Build history of the part. All positions in model axes, mm. A direction names the side the tool comes from. Give positions to 0.01 mm unless a question says otherwise; leave off trailing zeros. Order: outer loops, then holes, each group sorted by start corner. A loop starts at its lowest first (then second) coordinate and runs counter-clockwise, first axis right, second up. Notation, with made-up numbers: (21, -4) - (37, -4) arc R19 cw to (37, 8) - close; hole circle Ø3 at (69.5, 15.25). An arc over 180 degrees is marked (long way). Use a Markdown table: item, result.
Autodesk Fusion 360 part; units mm, degrees
sketch "スケッチ1" plane through (0, 0, 0) normal (0, 0, 1) x (1, 0, 0)
  line L0 (-9.5, 140) -> (-80.5, 140)
  line L1 (-80.5, 140) -> (-80.5, -140)
  line L2 (-80.5, -140) -> (-9.5, -140)
  line L3 (80.5, 20) -> (80.5, 130)
  line L4 (74.75, 130) -> (-80.5, -140) construction
  line L5 (-80.5, 140) -> (38.0073, -66.0997) construction
  line L6 (-9.5, 140) -> (-9.5, 130)
  line L7 (-9.5, 130) -> (80.5, 130)
  line L8 (-80.5, -140) -> (-9.5, -140) construction
  line L9 (80.5, 0) -> (-9.5, -140)
  line L10 (80.5, 0) -> (-9.5, 0)
  line L11 (-9.5, 0) -> (-9.5, 20)
  line L12 (-9.5, 20) -> (80.5, 20)
  dimension "d2" = 280
  dimension "d5" = 71
  dimension "d7" = 90
  dimension "d8" = 20
extrude "押し出し1" add sketch "スケッチ1" along normal blind 6
chamfer "面取り1" distance 25 angle 45 2 edges at (-80.5, -140, 3) (-80.5, 140, 3)
sketch "スケッチ2" plane through (0, 0, 6) normal (0, 0, 1) x (-1, 0, 0)
  line L0 (55.5, -140) -> (80.5, -115)
  line L1 (80.5, -115) -> (80.5, 115)
  line L2 (80.5, 115) -> (55.5, 140)
  line L3 (55.5, 140) -> (9.5, 140)
  line L4 (9.5, 140) -> (-80.5, 0)
  line L5 (-80.5, 0) -> (9.5, 0)
  line L6 (9.5, 0) -> (9.5, -20)
  line L7 (9.5, -20) -> (-80.5, -20)
  line L8 (-80.5, -20) -> (-80.5, -130)
  line L9 (-80.5, -130) -> (9.5, -130)
  line L10 (9.5, -130) -> (9.5, -140)
  line L11 (9.5, -140) -> (55.5, -140)
  line L12 (-80.5, -130) -> (-40.5, -130) construction
  line L13 (-40.5, -130) -> (-40.5, -100) construction
  line L14 (-40.5, -100) -> (-80.5, -100) construction
  line L15 (-80.5, -100) -> (-80.5, -130) construction
  line L16 (-40.5, -100) -> (-40.5, -50) construction
  point P0 (-40.5, -100)
  point P1 (-40.5, -50)
  dimension "d12" = 40
  dimension "d13" = 30
  dimension "d14" = 50
hole "穴1" at (40.5, 100, 6) at (40.5, 50, 6) direction (0, 0, -1) diameter 18 end through all
equation "d5 = 25 mm + 46 mm"
1) Slice it at A-A (y = 50). Write the cut outline in (x, z), and give its area (3 significant figures).
Computed:
| item | result |
|---|---|
| outline | (-80.5, 0) - (31.5, 0) - (31.5, 6) - (-80.5, 6) - close; (49.5, 0) - (80.5, 0) - (80.5, 6) - (49.5, 6) - close |
| area | 858 mm² |
2) Slice it at C-C (z = 4.9). Write the cut outline in (x, y), and give its area (3 significant figures).
Computed:
| item | result |
|---|---|
| outline | (-80.5, -115) - (-55.5, -140) - (-9.5, -140) - (80.5, 0) - (-9.5, 0) - (-9.5, 20) - (80.5, 20) - (80.5, 130) - (-9.5, 130) - (-9.5, 140) - (-55.5, 140) - (-80.5, 115) - close; hole circle Ø18 at (40.5, 50); hole circle Ø18 at (40.5, 100) |
| area | 34,900 mm² |
3) Slice it at B-B (x = 5). Write the cut outline in (y, z).
Computed:
| item | result |
|---|---|
| outline | (-117.44, 0) - (0, 0) - (0, 6) - (-117.44, 6) - close; (20, 0) - (130, 0) - (130, 6) - (20, 6) - close |
4) Two-plate mould, pull along X, no slides. Class faces 4 (the cylindrical face through (34.417, 56.633, 2.958)), 5 (the flat face through (-9.5, 10, 3)), 6 (the flat face through (35, 130, 3)): +X half, -X half, draft (parallel to the pull), parting line (faces both ways), or undercut.
Computed:
| item | result |
|---|---|
| face 4 | undercut |
| face 5 | +X half |
| face 6 | draft |
5) Pin check, flat tips, straight feed: P1, Ø3, axis at x = 21.5, z = 1.5, coming from the +Y side; P2, Ø3, axis at y = 10.5, z = 2, coming from the +X side. Stop position of each tip, or through.
Computed:
| item | result |
|---|---|
| P1 | stops at y = 130 |
| P2 | stops at x = -9.5 |
6) Slice it at D-D (x = 44). Write the cut outline in (y, z), and give its area (3 significant figures).
Computed:
| item | result |
|---|---|
| outline | (-56.78, 0) - (0, 0) - (0, 6) - (-56.78, 6) - close; (20, 0) - (41.71, 0) - (41.71, 6) - (20, 6) - close; (58.29, 0) - (91.71, 0) - (91.71, 6) - (58.29, 6) - close; (108.29, 0) - (130, 0) - (130, 6) - (108.29, 6) - close |
| area | 802 mm² |
7) Tool access for faces 1 (the flat face through (35, 20, 3)), 2 (the flat face through (-9.5, 135, 3)), 3 (the flat face through (80.5, 74, 3)): list every direction of +Z, -Z, +X, -X, +Y, -Y with a clear straight run to the whole face (end or side of a thin tool).
Computed:
| item | result |
|---|---|
| face 1 | +Z, -Z, +X |
| face 2 | +Z, -Z, +X, +Y |
| face 3 | +Z, -Z, +X, +Y, -Y |
8) Wall check: line 1 (X direction, y = 100, z = 4.2); line 2 (Y direction, x = 40.5, z = 3.55); line 3 (X direction, y = 94, z = 4.9). Give the ranges that are in metal, low to high. Write a range as from..to.
Computed:
| item | result |
|---|---|
| line 1 | x = -80.5..31.5, 49.5..80.5 |
| line 2 | y = -62.22..0, 20..41, 59..91, 109..130 |
| line 3 | x = -80.5..33.79, 47.21..80.5 |
